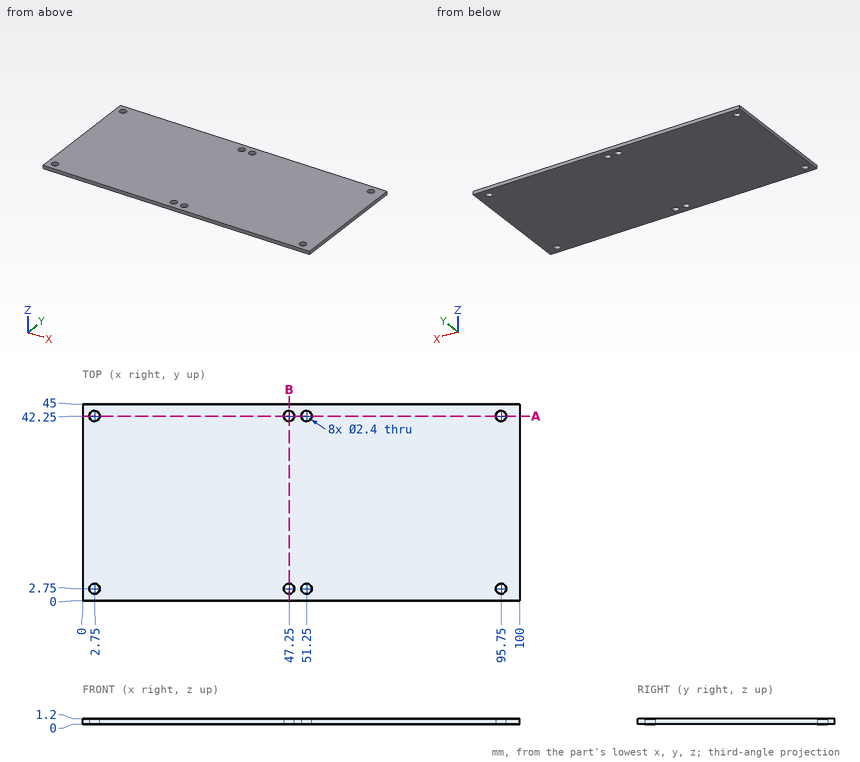
Can you work these out from the drawing? Everything is in mm from the part's minimum corner. Round coordinates to 2 decimals unless told otherwise and drop trailing zeros. Order: outer loops, then holes, each group sorted by start corner. A loop starts at its lowest first (then second) coordinate and runs counter-clockwise, first axis right, second up. Notation, with made-up numbers: (10.5, 77) -> (59.5, 77) arc R12 cw to (59.5, 96) -> close; hole circle Ø3 at (84.5, 12.25). An arc over 180 degrees is marked (long way). Return JSON: item names as keys, results as strings. Group by question number.
1. If we section it at A-A, the plane y = 42.25: Write out the boundary of the cut face in (x, z), then the cut area to 3 significant figures.
2. Will these pins go through, and if not, where does the flat tip stop? pin 1 (3 mm diameter, centred on x = 2.75, y = 2.75, fed in from +Z); pin 2 (1.4 mm diameter, centred on x = 51.25, y = 42.25, fed in from +Z).
3. I need wall thicknesses on line 1 (Y direction, x = 2.75, z = 0.8); line 2 (X direction, y = 42.25, z = 0.4). Which ranges of each line are inside material? Lowest first, please. Write a range as [from, to].
4. If we section it at B-B, the plane x = 47.25: Write out the boundary of the cut face in (y, z).
Output values:
{
 "1": {"outline": "(0, 0) -> (1.55, 0) -> (1.55, 1.2) -> (0, 1.2) -> close; (3.95, 0) -> (46.05, 0) -> (46.05, 1.2) -> (3.95, 1.2) -> close; (48.45, 0) -> (50.05, 0) -> (50.05, 1.2) -> (48.45, 1.2) -> close; (52.45, 0) -> (94.55, 0) -> (94.55, 1.2) -> (52.45, 1.2) -> close; (96.95, 0) -> (100, 0) -> (100, 1.2) -> (96.95, 1.2) -> close", "area": "108 mm²"},
 "2": {"pin 1": "z = 1.2", "pin 2": "through"},
 "3": {"line 1": "[0, 1.55], [3.95, 41.05], [43.45, 45]", "line 2": "[0, 1.55], [3.95, 46.05], [48.45, 50.05], [52.45, 94.55], [96.95, 100]"},
 "4": {"outline": "(0, 0) -> (1.55, 0) -> (1.55, 1.2) -> (0, 1.2) -> close; (3.95, 0) -> (41.05, 0) -> (41.05, 1.2) -> (3.95, 1.2) -> close; (43.45, 0) -> (45, 0) -> (45, 1.2) -> (43.45, 1.2) -> close"}
}
